from build123d import *

# Parameters (mm, degrees)
F0_R     = 11.425
F1_DEPTH = 8


with BuildPart() as f1:
    # F0 (on Top) → F1 (new body)
    with BuildSketch(Plane.XY):
        with BuildLine():
            ThreePointArc((-50.2454332161, 2.5664754466), (-52.4174873095, 22.6356659226), (-34.5842170537, 13.1770879466))
            ThreePointArc((-34.5842170537, 13.1770879466), (-36.5506390777, 6.7688176907), (-41.7730008912, 2.5664754466))
            ThreePointArc((-41.7730008912, 2.5664754466), (-40.0995641696, 1.963893334), (-38.5092170537, 1.1674690033))
            Line((-38.5092170537, 1.1674690033), (-31.0092170537, -3.1626580156))
            Line((-31.0092170537, -3.1626580156), (-31.0092170537, 13.1770879466))
            ThreePointArc((-31.0092170537, 13.1770879466), (-46.0092170537, 28.1770879466), (-61.0092170537, 13.1770879466))
            Line((-61.0092170537, 13.1770879466), (-61.0092170537, -3.1626580156))
            Line((-61.0092170537, -3.1626580156), (-53.5092170537, 1.1674690033))
            ThreePointArc((-53.5092170537, 1.1674690033), (-51.9188699377, 1.963893334), (-50.2454332161, 2.5664754466))
        make_face()
        with BuildLine():
            ThreePointArc((-61.0092170537, -11.8229120534), (-58.9995981104, -4.3229120534), (-53.5092170537, 1.1674690033))
            Line((-53.5092170537, 1.1674690033), (-61.0092170537, -3.1626580156))
            Line((-61.0092170537, -3.1626580156), (-61.0092170537, -11.8229120534))
        make_face()
        with BuildLine():
            Line((-31.0092170537, -3.1626580156), (-38.5092170537, 1.1674690033))
            ThreePointArc((-38.5092170537, 1.1674690033), (-33.0188359969, -4.3229120534), (-31.0092170537, -11.8229120534))
            Line((-31.0092170537, -11.8229120534), (-31.0092170537, -3.1626580156))
        make_face()
        with BuildLine():
            Line((-61.0092170537, -11.8229120534), (-61.0092170537, -3.1626580156))
            Line((-61.0092170537, -3.1626580156), (-75.1598521483, -11.3325309967))
            ThreePointArc((-75.1598521483, -11.3325309967), (-80.650233205, -31.8229120534), (-60.1598521483, -37.3132931102))
            Line((-60.1598521483, -37.3132931102), (-46.0092170537, -29.1434201291))
            Line((-46.0092170537, -29.1434201291), (-53.5092170537, -24.8132931102))
            ThreePointArc((-53.5092170537, -24.8132931102), (-54.9941143142, -23.8342242723), (-56.3526840923, -22.686276616))
            ThreePointArc((-56.3526840923, -22.686276616), (-56.2643482095, -23.5024762055), (-56.2348521483, -24.3229120534))
            ThreePointArc((-56.2348521483, -24.3229120534), (-77.9388659721, -29.3101457364), (-60.5889002548, -15.3489349908))
            ThreePointArc((-60.5889002548, -15.3489349908), (-60.9037671982, -13.598405222), (-61.0092170537, -11.8229120534))
        make_face()
        with BuildLine():
            Line((-31.0092170537, -3.1626580156), (-31.0092170537, -11.8229120534))
            ThreePointArc((-31.0092170537, -11.8229120534), (-31.1146669091, -13.598405222), (-31.4295338525, -15.3489349908))
            ThreePointArc((-31.4295338525, -15.3489349908), (-19.3713482761, -14.0438982295), (-12.933581959, -24.3229120534))
            ThreePointArc((-12.933581959, -24.3229120534), (-25.1790178069, -35.7184159922), (-35.665750015, -22.686276616))
            ThreePointArc((-35.665750015, -22.686276616), (-37.0243197932, -23.8342242723), (-38.5092170537, -24.8132931102))
            Line((-38.5092170537, -24.8132931102), (-46.0092170537, -29.1434201291))
            Line((-46.0092170537, -29.1434201291), (-31.858581959, -37.3132931102))
            ThreePointArc((-31.858581959, -37.3132931102), (-11.3682009023, -31.8229120534), (-16.858581959, -11.3325309967))
            Line((-16.858581959, -11.3325309967), (-31.0092170537, -3.1626580156))
        make_face()
        with BuildLine():
            Line((-53.5092170537, -24.8132931102), (-46.0092170537, -29.1434201291))
            Line((-46.0092170537, -29.1434201291), (-38.5092170537, -24.8132931102))
            ThreePointArc((-38.5092170537, -24.8132931102), (-46.0092170537, -26.8229120534), (-53.5092170537, -24.8132931102))
        make_face()
        with BuildLine():
            ThreePointArc((-41.7730008912, 2.5664754466), (-46.0092170537, 1.7520879466), (-50.2454332161, 2.5664754466))
            ThreePointArc((-50.2454332161, 2.5664754466), (-51.9188699377, 1.963893334), (-53.5092170537, 1.1674690033))
            ThreePointArc((-53.5092170537, 1.1674690033), (-58.9995981104, -4.3229120534), (-61.0092170537, -11.8229120534))
            ThreePointArc((-61.0092170537, -11.8229120534), (-60.9037671982, -13.598405222), (-60.5889002548, -15.3489349908))
            ThreePointArc((-60.5889002548, -15.3489349908), (-57.76551191, -18.6104120534), (-56.3526840923, -22.686276616))
            ThreePointArc((-56.3526840923, -22.686276616), (-54.9941143142, -23.8342242723), (-53.5092170537, -24.8132931102))
            ThreePointArc((-53.5092170537, -24.8132931102), (-46.0092170537, -26.8229120534), (-38.5092170537, -24.8132931102))
            ThreePointArc((-38.5092170537, -24.8132931102), (-37.0243197932, -23.8342242723), (-35.665750015, -22.686276616))
            ThreePointArc((-35.665750015, -22.686276616), (-34.2529221973, -18.6104120534), (-31.4295338525, -15.3489349908))
            ThreePointArc((-31.4295338525, -15.3489349908), (-31.1146669091, -13.598405222), (-31.0092170537, -11.8229120534))
            ThreePointArc((-31.0092170537, -11.8229120534), (-33.0188359969, -4.3229120534), (-38.5092170537, 1.1674690033))
            ThreePointArc((-38.5092170537, 1.1674690033), (-40.0995641696, 1.963893334), (-41.7730008912, 2.5664754466))
        make_face()
        with Locations((-46.0092170537, -11.8229120534)):
            Circle(F0_R, mode=Mode.SUBTRACT)
    extrude(amount=F1_DEPTH)


solid = f1.part
Could you check a few things on this model? Use its own coordinates, in mm. A direction names the side the tool comes from. Give positions to 0.01 mm unless a question says otherwise; leave off trailing zeros. Order: outer loops, then holes, each group sorted by start corner. A loop starts at its lowest first (then second) coordinate and runs counter-clockwise, first axis right, second up.
1. Suppose I cut it at D-D (y = 9). List the corners of the cut face in (x, z) for me.
2. Suppose I cut it at A-A (x = -72.5). List the corners of the cut face in (y, z) for me.
3. Suppose I cut it at B-B (y = -17). List the corners of the cut face in (x, z) for me, plus the area to 3 significant figures.
4. I need wall thicknesses on L1, parallel to Y at x = -46, z = 0.5; L2, parallel to Y at x = -53, z = 5.25; L3, parallel to X at y = -26.5, z = 6.5. Which ranges of each line are inside material? Lowest first, please.
5. We'd pull the mould along X, two halves only. Please class faces 1 (the flat face through (-53.184, -33.286, 3.944)), 2 (the flat face through (-57.04, -15.42, 8)), 3 (the flat face through (-31.009, 5, 4)), 4 (the flat face through (-68, -7.2, 3.9)): pulls with the +X half, pulls with the -X half, needs draft (parallel to the pull), parting line crosses it, or undercut.
6. Will these pins go through, and if not, where does the flat tip stop? P1, Ø3, axis at y = -29, z = 5.5, coming from the -X side; P2, Ø13.5, axis at x = -46.01, y = -11.82, coming from the +Z side; P3, Ø2, axis at y = 17.5, z = 4, coming from the +X side.
7. For faces 5 (the flat face through (-23.835, -7.305, 3.944)), 6 (the flat face through (-61.009, 5, 4)), 7 (the flat face through (-39.033, -33.171, 3.944)), which set-ups out of +Z, -Z, +X, -X, +Y, -Y let a thin tool reach every point of the face, with its end or its side?
Solved:
1. outline: (-61.01, 0) - (-56.64, 0) - (-56.64, 8) - (-61.01, 8) - close; (-35.38, 0) - (-31.01, 0) - (-31.01, 8) - (-35.38, 8) - close
2. outline: (-38.52, 0) - (-34.67, 0) - (-34.67, 8) - (-38.52, 8) - close; (-13.97, 0) - (-9.8, 0) - (-9.8, 8) - (-13.97, 8) - close
3. outline: (-80.75, 0) - (-76.43, 0) - (-76.43, 8) - (-80.75, 8) - close; (-58.89, 0) - (-56.19, 0) - (-56.19, 8) - (-58.89, 8) - close; (-35.82, 0) - (-33.13, 0) - (-33.13, 8) - (-35.82, 8) - close; (-15.59, 0) - (-11.27, 0) - (-11.27, 8) - (-15.59, 8) - close
3. area: 112 mm2
4. L1: y = -29.15 to -23.25, -0.4 to 1.75, 24.6 to 28.18
4. L2: y = -33.18 to -20.86, -2.79 to 4.14, 22.21 to 26.45
4. L3: x = -82.5 to -78.88, -56.44 to -35.57, -13.14 to -9.52
5. face 1: undercut
5. face 2: needs draft
5. face 3: pulls with the +X half
5. face 4: pulls with the -X half
6. P1: stops at x = -82.32
6. P2: passes through
6. P3: stops at x = -31.38
7. face 5: +Z, -Z, +X, +Y
7. face 6: +Z, -Z, -X, +Y
7. face 7: +Z, -Z, -Y
